```python
from build123d import *

# Parameters (mm, degrees)
BOSS_EXTRUDE1_DEPTH          = 19.05
FILLET1_R                    = 1.143
FILLET2_R                    = 0.762
FILLET3_R                    = 0.381
SKETCH4_R                    = 2.0828
CUT_EXTRUDE1_DEPTH           = 1.524
CUT_EXTRUDE1_DRAFT           = -41
CUT_EXTRUDE1_PROFILE_2_DEPTH = 1.524
CUT_EXTRUDE1_PROFILE_2_DRAFT = -41
CUT_EXTRUDE1_PROFILE_3_DEPTH = 1.524
CUT_EXTRUDE1_PROFILE_3_DRAFT = -41
SKETCH5_R                    = 2.0828
CUT_EXTRUDE2_DEPTH           = 1.524
CUT_EXTRUDE2_DRAFT           = -41
CUT_EXTRUDE2_PROFILE_2_DEPTH = 1.524
CUT_EXTRUDE2_PROFILE_2_DRAFT = -41
CUT_EXTRUDE2_PROFILE_3_DEPTH = 1.524
CUT_EXTRUDE2_PROFILE_3_DRAFT = -41


with BuildPart() as part:
    # Sketch3 → Boss-Extrude1 (new, symmetric)
    with BuildSketch(Plane(origin=(0, 0, 0), x_dir=(1, 0, 0), z_dir=(0, 1, 0))):
        Polygon((0.762, -0.762), (37.338, -0.762), (37.338, 0.762), (-0.762, 0.762), (-0.762, -37.338), (0.762, -37.338), align=None)
    extrude(amount=BOSS_EXTRUDE1_DEPTH, both=True)

    # Fillet1
    fillet1_edges = [part.edges().sort_by_distance(p)[0] for p in [
        (-0.762, 0, -0.762),
    ]]
    fillet(fillet1_edges, radius=FILLET1_R)

    # Fillet2
    fillet2_edges = [part.edges().sort_by_distance(p)[0] for p in [
        (0.762, 0, 0.762),
    ]]
    fillet(fillet2_edges, radius=FILLET2_R)

    # Fillet3
    fillet3_edges = [part.edges().sort_by_distance(p)[0] for p in [
        (37.338, 19.05, 0),
        (0, 19.05, 37.338),
        (0, -19.05, 37.338),
        (37.338, -19.05, 0),
    ]]
    fillet(fillet3_edges, radius=FILLET3_R)


with BuildPart() as cut_extrude1_tool:
    # Sketch4 → Cut-Extrude1 (with draft: the straight prism first)
    with BuildSketch(Plane(origin=(-0.762, 0, 0), x_dir=(0, 0, -1), z_dir=(1, 0, 0))):
        with Locations((-27.813, 0)):
            Circle(SKETCH4_R)
    extrude(amount=CUT_EXTRUDE1_DEPTH)
    # Cut-Extrude1: the draft: its side faces are tilted about the plane it starts from
    cut_extrude1_sides = [cut_extrude1_tool.faces().sort_by_distance(p)[0] for p in [
        (0, 0, 29.8958),
    ]]
    draft(cut_extrude1_sides, Plane(origin=(-0.762, 0, 0), x_dir=(0, 0, -1), z_dir=(1, 0, 0)), CUT_EXTRUDE1_DRAFT)


with BuildPart() as part_1:
    add(part.part)

    # Cut-Extrude1: cut by cut_extrude1_tool
    add(cut_extrude1_tool.part, mode=Mode.SUBTRACT)


with BuildPart() as cut_extrude1_profile_2_tool:
    # Sketch4 → Cut-Extrude1 profile 2 (with draft: the straight prism first)
    with BuildSketch(Plane(origin=(-0.762, 0, 0), x_dir=(0, 0, -1), z_dir=(1, 0, 0))):
        with Locations((-13.5128, 12.7)):
            Circle(SKETCH4_R)
    extrude(amount=CUT_EXTRUDE1_PROFILE_2_DEPTH)
    # Cut-Extrude1 profile 2: the draft: its side faces are tilted about the plane it starts from
    cut_extrude1_profile_2_sides = [cut_extrude1_profile_2_tool.faces().sort_by_distance(p)[0] for p in [
        (0, 12.7, 15.5956),
    ]]
    draft(cut_extrude1_profile_2_sides, Plane(origin=(-0.762, 0, 0), x_dir=(0, 0, -1), z_dir=(1, 0, 0)), CUT_EXTRUDE1_PROFILE_2_DRAFT)


with BuildPart() as part_2:
    add(part_1.part)

    # Cut-Extrude1 profile 2: cut by cut_extrude1_profile_2_tool
    add(cut_extrude1_profile_2_tool.part, mode=Mode.SUBTRACT)


with BuildPart() as cut_extrude1_profile_3_tool:
    # Sketch4 → Cut-Extrude1 profile 3 (with draft: the straight prism first)
    with BuildSketch(Plane(origin=(-0.762, 0, 0), x_dir=(0, 0, -1), z_dir=(1, 0, 0))):
        with Locations((-13.5128, -12.7)):
            Circle(SKETCH4_R)
    extrude(amount=CUT_EXTRUDE1_PROFILE_3_DEPTH)
    # Cut-Extrude1 profile 3: the draft: its side faces are tilted about the plane it starts from
    cut_extrude1_profile_3_sides = [cut_extrude1_profile_3_tool.faces().sort_by_distance(p)[0] for p in [
        (0, -12.7, 15.5956),
    ]]
    draft(cut_extrude1_profile_3_sides, Plane(origin=(-0.762, 0, 0), x_dir=(0, 0, -1), z_dir=(1, 0, 0)), CUT_EXTRUDE1_PROFILE_3_DRAFT)


with BuildPart() as part_3:
    add(part_2.part)

    # Cut-Extrude1 profile 3: cut by cut_extrude1_profile_3_tool
    add(cut_extrude1_profile_3_tool.part, mode=Mode.SUBTRACT)


with BuildPart() as cut_extrude2_tool:
    # Sketch5 → Cut-Extrude2 (with draft: the straight prism first)
    with BuildSketch(Plane.XY.offset(-0.762)):
        with Locations((13.5128, 12.7)):
            Circle(SKETCH5_R)
    extrude(amount=CUT_EXTRUDE2_DEPTH)
    # Cut-Extrude2: the draft: its side faces are tilted about the plane it starts from
    cut_extrude2_sides = [cut_extrude2_tool.faces().sort_by_distance(p)[0] for p in [
        (11.43, 12.7, 0),
    ]]
    draft(cut_extrude2_sides, Plane.XY.offset(-0.762), CUT_EXTRUDE2_DRAFT)


with BuildPart() as part_4:
    add(part_3.part)

    # Cut-Extrude2: cut by cut_extrude2_tool
    add(cut_extrude2_tool.part, mode=Mode.SUBTRACT)


with BuildPart() as cut_extrude2_profile_2_tool:
    # Sketch5 → Cut-Extrude2 profile 2 (with draft: the straight prism first)
    with BuildSketch(Plane.XY.offset(-0.762)):
        with Locations((13.5128, -12.7)):
            Circle(SKETCH5_R)
    extrude(amount=CUT_EXTRUDE2_PROFILE_2_DEPTH)
    # Cut-Extrude2 profile 2: the draft: its side faces are tilted about the plane it starts from
    cut_extrude2_profile_2_sides = [cut_extrude2_profile_2_tool.faces().sort_by_distance(p)[0] for p in [
        (11.43, -12.7, 0),
    ]]
    draft(cut_extrude2_profile_2_sides, Plane.XY.offset(-0.762), CUT_EXTRUDE2_PROFILE_2_DRAFT)


with BuildPart() as part_5:
    add(part_4.part)

    # Cut-Extrude2 profile 2: cut by cut_extrude2_profile_2_tool
    add(cut_extrude2_profile_2_tool.part, mode=Mode.SUBTRACT)


with BuildPart() as cut_extrude2_profile_3_tool:
    # Sketch5 → Cut-Extrude2 profile 3 (with draft: the straight prism first)
    with BuildSketch(Plane.XY.offset(-0.762)):
        with Locations((27.813, 0)):
            Circle(SKETCH5_R)
    extrude(amount=CUT_EXTRUDE2_PROFILE_3_DEPTH)
    # Cut-Extrude2 profile 3: the draft: its side faces are tilted about the plane it starts from
    cut_extrude2_profile_3_sides = [cut_extrude2_profile_3_tool.faces().sort_by_distance(p)[0] for p in [
        (25.7302, 0, 0),
    ]]
    draft(cut_extrude2_profile_3_sides, Plane.XY.offset(-0.762), CUT_EXTRUDE2_PROFILE_3_DRAFT)


with BuildPart() as part_6:
    add(part_5.part)

    # Cut-Extrude2 profile 3: cut by cut_extrude2_profile_3_tool
    add(cut_extrude2_profile_3_tool.part, mode=Mode.SUBTRACT)


solid = part_6.part
```
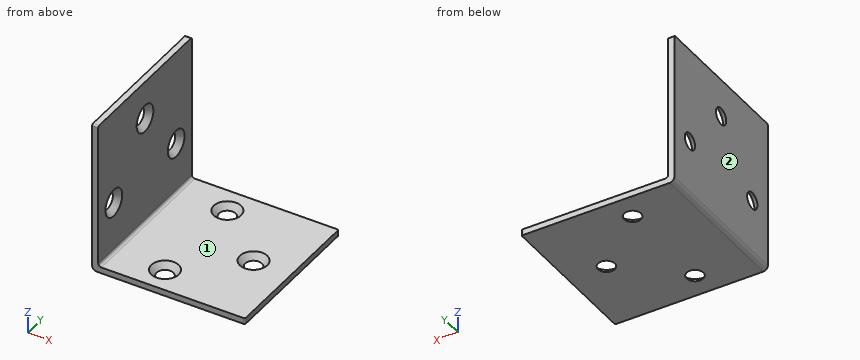
Geometry: final body of the model. Coordinates: model frame, mm. Face numbers are marked on the shaded views. A direction names the side the tool comes from. Give positions to 0.01 mm unless a question says otherwise; leave off trailing zeros. Order: outer loops, then holes, each group sorted by start corner. A loop starts at its lowest first (then second) coordinate and runs counter-clockwise, first axis right, second up. Notation, with made-up numbers: (60, 74) -> (66, 74) arc R21 ccw to (66, 93) -> close; hole circle Ø6 at (-23.5, -19.75). An arc over 180 degrees is marked (long way). Write each question's results on one line, items separated by ' | '. Start each with the question number.
1) Set-up query: the marked faces 1 and 2. Return all of +Z, -Z, +X, -X, +Y, -Y with unobstructed straight access to the full face (end or side cutting, diameter ignored); none if empty.
2) Section D-D (z = 8). Return loops of the section in (x, y), then the cut area to 3 significant figures.
3) First-contact query: pin 1 (12 mm diameter, centred on y = 0.5, z = 30, fed in from +X); pin 2 (4 mm diameter, centred on x = 7.5, y = 13.5, fed in from +Z). Flat tips, straight axial feed; report the tip coordinate or a pass-through.
4) Section C-C (x = 12). Count the separate pieces of the cut face and the enclosed holes in it, then the cut area to 3 significant figures.
5) Section A-A (y = 0). Return loops of the section in (x, z).
6) Section B-B (y = 7). Return loops of the section in (x, z).
7) Line query: line 1 (X direction, y = 11, z = 2); line 2 (Z direction, x = 14, y = -10.5). Output: solid intervals per line, ascending. Write a range as from..to.
Calculated:
1) face 1: +Z, +X, +Y, -Y | face 2: +Z, -Z, -X, +Y, -Y
2) outline: (-0.76, -19.05) -> (0.76, -19.05) -> (0.76, 19.05) -> (-0.76, 19.05) -> close | area: 58.1 mm2
3) pin 1: x = 0.76 | pin 2: z = 0.76
4) separate pieces: 3 | enclosed holes: 0 | area: 44.2 mm2
5) outline: (-0.76, 0.38) arc R1.14 ccw to (0.38, -0.76) -> (25.73, -0.76) -> (24.41, 0.76) -> (1.52, 0.76) arc R0.76 cw to (0.76, 1.52) -> (0.76, 24.41) -> (-0.76, 25.73) -> close; (-0.76, 29.9) -> (0.76, 31.22) -> (0.76, 37.34) -> (-0.76, 37.34) -> close; (29.9, -0.76) -> (37.34, -0.76) -> (37.34, 0.76) -> (31.22, 0.76) -> close
6) outline: (-0.76, 0.38) arc R1.14 ccw to (0.38, -0.76) -> (37.34, -0.76) -> (37.34, 0.76) -> (1.52, 0.76) arc R0.76 cw to (0.76, 1.52) -> (0.76, 37.34) -> (-0.76, 37.34) -> close
7) line 1: -0.76..0.76 | line 2: -0.76..-0.57
